Part model, mm, in its own coordinate system. Round coordinates to 2 decimals unless told otherwise and drop trailing zeros. Write each loop counter-clockwise with the first axis right and the second up, starting at its lowest first coordinate (ties: lowest second). Pieces come first, ordered by that corner, then holes.
1) Flat gauge pins, fed straight in: pin 1 (1.6 mm diameter, centred on x = 2.5, z = -1.5, fed in from +Y); pin 2 (3 mm diameter, centred on y = -7.5, z = -4.5, fed in from -X); pin 3 (1.5 mm diameter, centred on y = -287.5, z = -3, fed in from +X). Where does each tip first touch, or does it go through?
2) Saw through at A-A on y = -167.5. Write the cut outline in (x, z).
3) Drill centre lines: L1, parallel to X at y = -33.5, z = -3.75; L2, parallel to X at y = -489, z = -4. Where is each one in solid material? Low to high.
Autodesk Inventor part; units mm, degrees
ref_plane "YZ Plane" through (0, 0, 0) normal (1, 0, 0) x (0, 1, 0)
ref_plane "XZ Plane" through (0, 0, 0) normal (0, 1, 0) x (-1, 0, 0)
ref_plane "XY Plane" through (0, 0, 0) normal (0, 0, 1) x (1, 0, 0)
sketch "Sketch1" plane through (0, 0, 0) normal (0, 0, 1) x (1, 0, 0)
  line L0 (0, 0) -> (0, 20)
  line L1 (79.3918, 0) -> (79.3918, 20)
  line L2 (79.3918, 0) -> (0, 0)
  line L3 (-0.2277, -520) -> (79.6269, -520)
  line L4 (5.4724, 0) -> (74.116, 0)
  line L5 (79.6269, -520) -> (0, -520)
  line L6 (74.116, -20) -> (74.116, 0)
  line L7 (74.116, 0) -> (74.116, -20)
  line L8 (74.116, -20) -> (79.5884, -20)
  line L9 (0, -20) -> (5.4724, -20)
  line L10 (5.4724, -20) -> (5.4724, 0)
  line L11 (39.7942, 0) -> (39.7942, -37.2544) construction
  line L12 (0, -20) -> (0, -40)
  line L13 (0, -40) -> (5.4724, -40)
  line L14 (79.5884, -20) -> (79.5884, -40)
  line L15 (79.5884, -40) -> (74.28, -40)
  line L16 (5.4724, -40) -> (5.4724, -60)
  line L17 (5.4724, -60) -> (0, -60)
  line L18 (0, -60) -> (0, -80)
  line L19 (0, -80) -> (5.4724, -80)
  line L20 (5.4724, -80) -> (5.4724, -100)
  line L21 (5.4724, -100) -> (0, -100)
  line L22 (0, -100) -> (0, -120)
  line L23 (0, -120) -> (5.4724, -120)
  line L24 (5.4724, -120) -> (5.4724, -140)
  line L25 (5.4724, -140) -> (0, -140)
  line L26 (0, -140) -> (0, -160)
  line L27 (0, -160) -> (5.4724, -160)
  line L28 (5.4724, -160) -> (5.4724, -180)
  line L29 (5.4724, -180) -> (0, -180)
  line L30 (0, -180) -> (0, -200)
  line L31 (0, -200) -> (5.4724, -200)
  line L32 (5.4724, -200) -> (5.4724, -220)
  line L33 (5.4724, -220) -> (0, -220)
  line L34 (0, -220) -> (0, -240)
  line L35 (0, -240) -> (5.4724, -240)
  line L36 (5.4724, -240) -> (5.4724, -260)
  line L37 (5.4724, -260) -> (0, -260)
  line L38 (0, -260) -> (0, -280)
  line L39 (0, -280) -> (5.4724, -280)
  line L40 (5.4724, -280) -> (5.4724, -300)
  line L41 (5.4724, -300) -> (0, -300)
  line L42 (0, -300) -> (0, -320)
  line L43 (0, -320) -> (5.4724, -320)
  line L44 (5.4724, -320) -> (5.4724, -340)
  line L45 (5.4724, -340) -> (0, -340)
  line L46 (0, -340) -> (0, -360)
  line L47 (0, -360) -> (5.4724, -360)
  line L48 (5.4724, -360) -> (5.4724, -380)
  line L49 (5.4724, -380) -> (0, -380)
  line L50 (0, -380) -> (0, -400)
  line L51 (0, -400) -> (5.4724, -400)
  line L52 (5.4724, -400) -> (5.4724, -420)
  line L53 (5.4724, -420) -> (0, -420)
  line L54 (0, -420) -> (0, -440)
  line L55 (0, -440) -> (5.4724, -440)
  line L56 (5.4724, -440) -> (5.4724, -460)
  line L57 (5.4724, -460) -> (0, -460)
  line L58 (0, -460) -> (0, -480)
  line L59 (0, -480) -> (5.4724, -480)
  line L60 (5.4724, -480) -> (5.4724, -500)
  line L61 (5.4724, -500) -> (0, -500)
  line L62 (0, -500) -> (0, -520)
  line L63 (74.28, -40) -> (74.28, -60)
  line L64 (74.28, -60) -> (79.6269, -60)
  line L65 (79.6269, -60) -> (79.6269, -80)
  line L66 (79.6269, -80) -> (74.28, -80)
  line L67 (74.28, -80) -> (74.28, -100)
  line L68 (74.28, -100) -> (79.6269, -100)
  line L69 (79.6269, -100) -> (79.6269, -120)
  line L70 (79.6269, -120) -> (74.28, -120)
  line L71 (74.28, -120) -> (74.28, -140)
  line L72 (74.28, -140) -> (79.6269, -140)
  line L73 (79.6269, -140) -> (79.6269, -160)
  line L74 (79.6269, -160) -> (74.28, -160)
  line L75 (74.28, -160) -> (74.28, -180)
  line L76 (74.28, -180) -> (79.6269, -180)
  line L77 (79.6269, -180) -> (79.6269, -200)
  line L78 (79.6269, -200) -> (74.28, -200)
  line L79 (74.28, -200) -> (74.28, -220)
  line L80 (74.28, -220) -> (79.6269, -220)
  line L81 (79.6269, -220) -> (79.6269, -240)
  line L82 (79.6269, -240) -> (74.28, -240)
  line L83 (74.28, -240) -> (74.28, -260)
  line L84 (74.28, -260) -> (79.6269, -260)
  line L85 (79.6269, -260) -> (79.6269, -280)
  line L86 (79.6269, -280) -> (74.28, -280)
  line L87 (74.28, -280) -> (74.28, -300)
  line L88 (74.28, -300) -> (79.6269, -300)
  line L89 (79.6269, -300) -> (79.6269, -320)
  line L90 (79.6269, -320) -> (74.28, -320)
  line L91 (74.28, -320) -> (74.28, -340)
  line L92 (74.28, -340) -> (79.6269, -340)
  line L93 (79.6269, -340) -> (79.6269, -360)
  line L94 (79.6269, -360) -> (74.28, -360)
  line L95 (74.28, -360) -> (74.28, -380)
  line L96 (74.28, -380) -> (79.6269, -380)
  line L97 (79.6269, -380) -> (79.6269, -400)
  line L98 (79.6269, -400) -> (74.28, -400)
  line L99 (74.28, -400) -> (74.28, -420)
  line L100 (74.28, -420) -> (79.6269, -420)
  line L101 (79.6269, -420) -> (79.6269, -440)
  line L102 (79.6269, -440) -> (74.28, -440)
  line L103 (74.28, -440) -> (74.28, -460)
  line L104 (74.28, -460) -> (79.6269, -460)
  line L105 (79.6269, -460) -> (79.6269, -480)
  line L106 (79.6269, -480) -> (74.28, -480)
  line L107 (74.28, -480) -> (74.28, -500)
  line L108 (74.28, -500) -> (79.6269, -500)
  line L109 (79.6269, -500) -> (79.6269, -520)
  dimension "d16" = 20
  dimension "d17" = 20
  dimension "d18" = 20
  dimension "d19" = 20
  dimension "d20" = 20
  dimension "d21" = 20
  dimension "d22" = 20
  dimension "d23" = 20
  dimension "d24" = 20
  dimension "d25" = 20
  dimension "d26" = 20
  dimension "d27" = 20
  dimension "d28" = 20
  dimension "d29" = 20
  dimension "d30" = 20
  dimension "d31" = 20
  dimension "d32" = 20
  dimension "d33" = 20
  dimension "d34" = 20
  dimension "d35" = 20
  dimension "d36" = 20
  dimension "d37" = 20
  dimension "d38" = 20
  dimension "d39" = 20
extrude "Extrusion1" add sketch "Sketch1" against normal blind 6.35
properties part number "small wall"
Completed:
1. pin 1: stops at y = -20
1. pin 2: stops at x = 5.47
1. pin 3: stops at x = 74.28
2. outline: (5.47, -6.35) - (74.28, -6.35) - (74.28, 0) - (5.47, 0) - close
3. L1: x = 0 to 79.59
3. L2: x = 5.47 to 74.28
